Study the drawing (mm; zero at the part's minimum x, y, z) and answer. A direction names the side the tool comes from. Coordinates: 2 decimals unless noted, no trailing zeros. Loops run counter-clockwise (first coordinate to the right, second up) from the corner with the lowest first, then second, coordinate; pieces in that order, holes last. Notation, with made-up numbers: (45.25, 79) -> (75.25, 79) arc R21 cw to (75.25, 111) -> close; hole circle Ø3 at (-40, -37). An arc over 180 degrees is marked (long way). Answer as a JSON object with one key per item and string values. Group by question number.
Q1. The part is cut by section A-A on z = 101.6. Write down the section's boundary in (x, y) (1 decimal), and give its area (3 significant figures).
Q2. For the marked faces 1, 2 and 3, determine the directions among +Z, -Z, +X, -X, +Y, -Y from which every point of the face is accessible in a straight line to the end or side of a thin tool.
Q3. Determine the mould class of the marked faces 4, 5 and 6 for opening direction X: released by +X, released by -X, zero draft, split by the parting line, or undercut.
Q4. The part is cut by section B-B on y = 9. Write down the section's boundary in (x, z) (1 decimal).
Q5. Each of these flat-tipped pins is pushed along its axis until it touches: P1, Ø8, axis at x = 49, y = 18.5, coming from the +Z side; P2, Ø16.5, axis at x = 31.75, z = 101.6, coming from the -Y side; P3, Ø4, axis at x = 48.5, z = 19, coming from the -Y side. Where does it stop, or does it pass through?
Q6. Straight lines are drawn through the part: line 1 along Z through (x, y) = (33, 9.5); line 2 along Y through (x, z) = (25, 73) (1 decimal); line 3 along Z through (x, y) = (26.5, 18). For each, find the intervals that lie inside material, in ascending order. Write a range as [from, to].
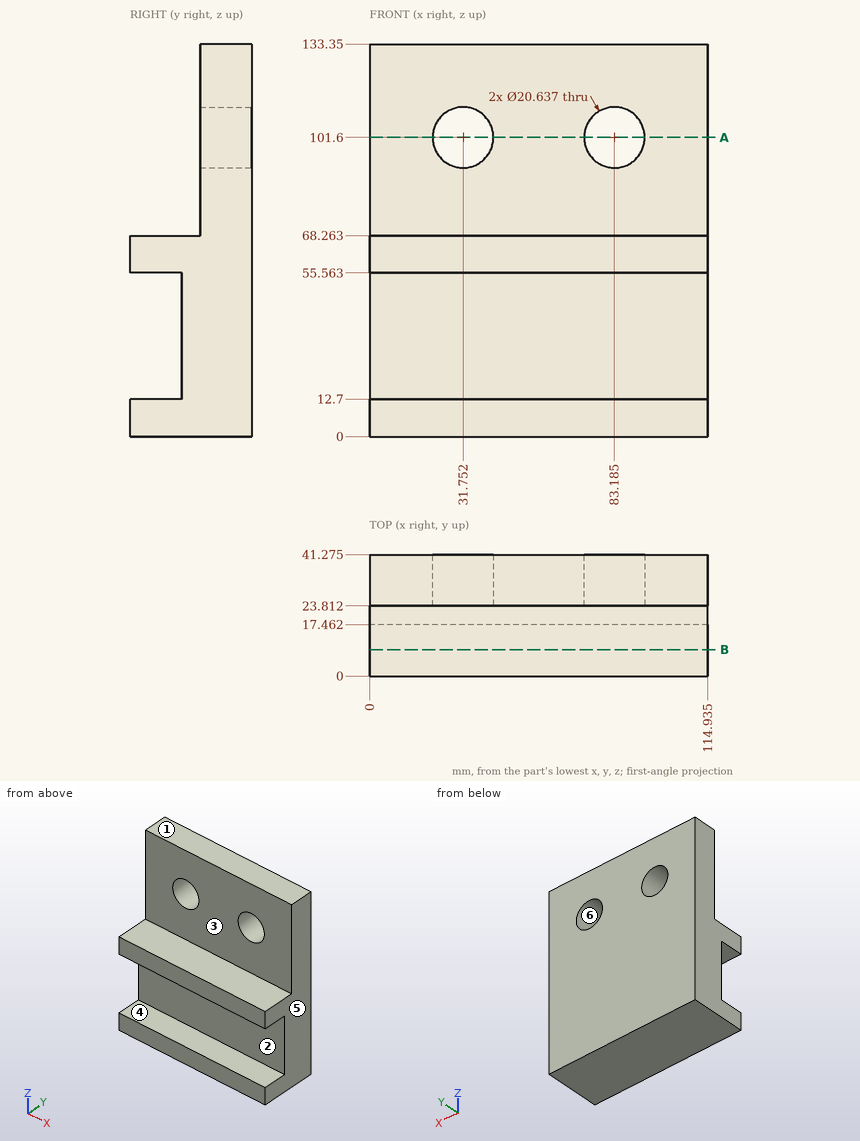
Final values:
{
 "1": {"outline": "(0, 23.8) -> (21.4, 23.8) -> (21.4, 41.3) -> (0, 41.3) -> close; (42.1, 23.8) -> (72.9, 23.8) -> (72.9, 41.3) -> (42.1, 41.3) -> close; (93.5, 23.8) -> (114.9, 23.8) -> (114.9, 41.3) -> (93.5, 41.3) -> close", "area": "1,290 mm2"},
 "2": {"face 1": "+Z, +X, -X, +Y, -Y", "face 2": "+X, -X, -Y", "face 3": "+Z, +X, -X, -Y"},
 "3": {"face 4": "zero draft", "face 5": "released by +X", "face 6": "undercut"},
 "4": {"outline": "(0, 0) -> (114.9, 0) -> (114.9, 12.7) -> (0, 12.7) -> close; (0, 55.6) -> (114.9, 55.6) -> (114.9, 68.3) -> (0, 68.3) -> close"},
 "5": {"P1": "stops at z = 68.26", "P2": "passes through", "P3": "stops at y = 17.46"},
 "6": {"line 1": "z = [0, 12.7], [55.56, 68.26]", "line 2": "y = [23.8, 41.3]", "line 3": "z = [0, 68.26]"}
}
